Work out the finished part from the listing and answer in its coordinate system (mm). A direction names the side the tool comes from. Round coordinates to 2 decimals unless told otherwise and drop trailing zeros. Loops run counter-clockwise (first coordinate to the right, second up) from the corner with the lowest first, then second, coordinate; pieces in that order, holes last.
```python
from build123d import *

# Parameters (mm, degrees)
SKETCH1_R          = 11.43
MAIN_BODY_DEPTH    = 6.35
NIBBLES_DEPTH      = 5.08
NIBBLES_DEPTH_BACK = 11.43
SKETCH13_R         = 2.54


with BuildPart() as part:
    # Sketch1 → main body (new body)
    with BuildSketch(Plane.XY):
        Circle(SKETCH1_R)
    extrude(amount=MAIN_BODY_DEPTH)

    # Sketch13 → nibbles (add, two sides: drawn at the far end of the back side and taken through both)
    with BuildSketch(Plane(origin=(0, 0, 0), x_dir=(-1, 0, 0), z_dir=(0, 0, -1)).offset(-NIBBLES_DEPTH_BACK)):
        Circle(SKETCH13_R)
    extrude(amount=NIBBLES_DEPTH + NIBBLES_DEPTH_BACK)


solid = part.part
```
1. Given pin 1 (2 mm diameter, centred on x = 7, y = 3.5, fed in from +Z); pin 2 (4 mm diameter, centred on x = 6, z = -1.5, fed in from +Y); pin 3 (6 mm diameter, centred on y = 5, z = 8.5, fed in from -X), each flat-ended and moving along its own axis, determine where each tip first touches the part or whether it passes through.
Answer key:
pin 1: stops at z = 6.35
pin 2: stops at y = 10.43
pin 3: stops at x = -11.05
2. Find section A-A (x = 0). Write down the section's boundary in (y, z).
Answer key:
outline: (-11.43, 0) - (-2.54, 0) - (-2.54, -5.08) - (2.54, -5.08) - (2.54, 0) - (11.43, 0) - (11.43, 6.35) - (2.54, 6.35) - (2.54, 11.43) - (-2.54, 11.43) - (-2.54, 6.35) - (-11.43, 6.35) - close
3. Which of the six approach directions +Z, -Z, +X, -X, +Y, -Y give full straight-line access (tool end or side, diameter ignored) to faces 1 (the face through (0.33, 2.52, -2.5)), 2 (the face through (0.33, 2.52, 8.93)), 3 (the face through (10.902, 3.433, 3.131))?
Answer key:
face 1: -Z
face 2: +Z
face 3: +Z, -Z
4. Find section D-D (z = 1.5). Write down the section's boundary in (x, y), then the cut area to 3 significant figures.
Answer key:
outline: circle Ø22.86 at (0, 0)
area: 410 mm2
5. Find section C-C (z = 9). Write down the section's boundary in (x, y).
Answer key:
outline: circle Ø5.08 at (0, 0)
6. Consider probe 1 along Z at (x, y) = (1.5, -8); probe 2 along Y at (x, z) = (0, 6); probe 3 along X at (y, z) = (1.5, -3.25). Determine where each line is inside the solid, lowest interval first.
Answer key:
probe 1: z = 0 to 6.35
probe 2: y = -11.43 to 11.43
probe 3: x = -2.05 to 2.05
